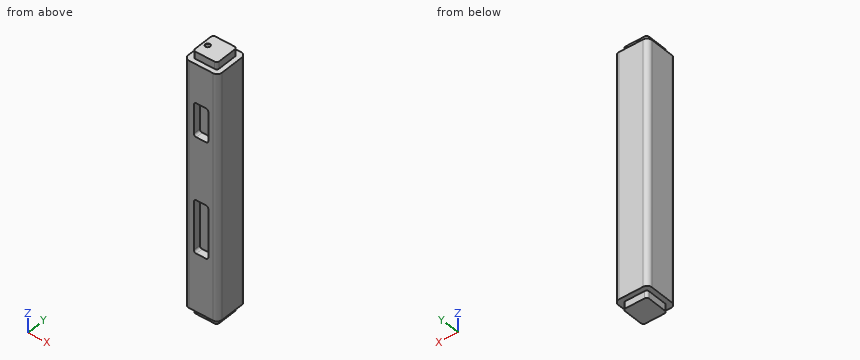
from build123d import *

# Parameters (mm, degrees)
F2_DEPTH  = 647.7
F4_DEPTH  = 19.05
F5_R      = 12.7
F6_R      = 6.35
F7_W      = 38.1
F7_H      = 139.7
F8_DEPTH  = 19.05
F9_R      = 6.35
F11_DEPTH = 19.05
F13_DEPTH = 19.05
F14_R     = 6.35
F15_DEPTH = 2.54


with BuildPart() as f2:
    # F1 (on Top) → F2 (new body)
    with BuildSketch(Plane.XY):
        Polygon((-44.45, 19.05), (-44.45, 0), (-44.45, -19.05), (-44.45, -44.45), (-19.05, -44.45), (0, -44.45), (19.05, -44.45), (44.45, -44.45), (44.45, -19.05), (44.45, 0), (44.45, 19.05), (44.45, 44.45), (19.05, 44.45), (0, 44.45), (-19.05, 44.45), (-44.45, 44.45), align=None)
    extrude(amount=-F2_DEPTH)

    # F3 (on face) → F4 (cut)
    with BuildSketch(Plane.XZ.offset(44.45)):
        Polygon((19.05, -101.6), (-19.05, -101.6), (-19.05, -190.5), (0, -190.5), (19.05, -190.5), align=None)
    extrude(amount=-F4_DEPTH, mode=Mode.SUBTRACT)

    # F5
    f5_edges = [f2.edges().sort_by_distance(p)[0] for p in [
        (-44.45, -44.45, -323.85),
        (44.45, -44.45, -323.85),
        (44.45, 44.45, -323.85),
        (-44.45, 44.45, -323.85),
    ]]
    fillet(f5_edges, radius=F5_R)

    # F6
    f6_edges = [f2.edges().sort_by_distance(p)[0] for p in [
        (-19.05, -34.925, -190.5),
        (19.05, -34.925, -190.5),
        (-19.05, -34.925, -101.6),
        (19.05, -34.925, -101.6),
    ]]
    fillet(f6_edges, radius=F6_R)

    # F7 (on face) → F8 (cut)
    with BuildSketch(Plane.XZ.offset(44.45)):
        with Locations((0, -425.45)):
            Rectangle(F7_W, F7_H)
    extrude(amount=-F8_DEPTH, mode=Mode.SUBTRACT)

    # F9
    f9_edges = [f2.edges().sort_by_distance(p)[0] for p in [
        (-19.05, -34.925, -355.6),
        (19.05, -34.925, -355.6),
        (19.05, -34.925, -495.3),
        (-19.05, -34.925, -495.3),
    ]]
    fillet(f9_edges, radius=F9_R)

    # F10 (on face) → F11 (join)
    with BuildSketch(Plane.XY):
        with BuildLine():
            Line((-25.4, -31.75), (25.4, -31.75))
            ThreePointArc((25.4, -31.75), (29.8901280605, -29.8901280605), (31.75, -25.4))
            Line((31.75, -25.4), (31.75, 25.4))
            ThreePointArc((31.75, 25.4), (29.8901280605, 29.8901280605), (25.4, 31.75))
            Line((25.4, 31.75), (-25.4, 31.75))
            ThreePointArc((-25.4, 31.75), (-29.8901280605, 29.8901280605), (-31.75, 25.4))
            Line((-31.75, 25.4), (-31.75, -25.4))
            ThreePointArc((-31.75, -25.4), (-29.8901280605, -29.8901280605), (-25.4, -31.75))
        make_face()
    extrude(amount=F11_DEPTH)

    # F12 (on face) → F13 (join)
    with BuildSketch(Plane(origin=(0, 0, -647.7), x_dir=(1, 0, 0), z_dir=(0, 0, -1))):
        with BuildLine():
            Line((-25.4, -31.75), (25.4, -31.75))
            ThreePointArc((25.4, -31.75), (29.8901280605, -29.8901280605), (31.75, -25.4))
            Line((31.75, -25.4), (31.75, 25.4))
            ThreePointArc((31.75, 25.4), (29.8901280605, 29.8901280605), (25.4, 31.75))
            Line((25.4, 31.75), (-25.4, 31.75))
            ThreePointArc((-25.4, 31.75), (-29.8901280605, 29.8901280605), (-31.75, 25.4))
            Line((-31.75, 25.4), (-31.75, -25.4))
            ThreePointArc((-31.75, -25.4), (-29.8901280605, -29.8901280605), (-25.4, -31.75))
        make_face()
    extrude(amount=F13_DEPTH)

    # F14 (on face) → F15 (cut)
    with BuildSketch(Plane.XY.offset(19.05)):
        with Locations((-19.05, 0)):
            Circle(F14_R)
    extrude(amount=-F15_DEPTH, mode=Mode.SUBTRACT)


solid = f2.part
Part model, mm, in its own coordinate system. Coordinates: 2 decimals unless noted, no trailing zeros. Loops run counter-clockwise (first coordinate to the right, second up) from the corner with the lowest first, then second, coordinate; pieces in that order, holes last. Notation, with made-up numbers: M 3.5,4.25 L 56.5,4.25 A23 ccw 56.5,38.25 Z; hole C 79.5,-23 d8. An arc over 180 degrees is marked long. Use a Markdown table: item, result. Add a question column.
Q1. Probe L1, parallel to Z at x = 8.5, y = -40; L2, parallel to Y at x = -19.05, z = 17; L3, parallel to Z at x = 31, y = -33. List the from-to ranges inside material, lowest first.
Q2. Cut at A-A (z = -572). Write the cut outline in (x, y), and give its area (3 significant figures).
Q3. Pin check, flat tips, straight feed: P1, Ø15, axis at x = 0, y = -36, coming from the -Z side; P2, Ø5.5, axis at x = 7, z = -660.5, coming from the +Y side; P3, Ø15, axis at x = -10.5, z = -659.5, coming from the -Y side; P4, Ø19, axis at x = -8.5, z = -133.5, coming from the -Y side. Stop position of each tip, or through.
Q4. Cut at D-D (z = -447). Write the cut outline in (x, y).
Q5. Cut at B-B (x = -1). Write the cut outline in (y, z).
Q6. Cut at C-C (y = 0). Write the cut outline in (x, z), and give its area (3 significant figures).
Worked out:
| question | item | result |
|---|---|---|
| 1 | L1 | z = -647.7 to -495.3, -355.6 to -190.5, -101.6 to 0 |
| 1 | L2 | y = -31.75 to -6.35, 6.35 to 31.75 |
| 1 | L3 | z = -647.7 to 0 |
| 2 | outline | M -44.45,-31.75 A12.7 ccw -31.75,-44.45 L 31.75,-44.45 A12.7 ccw 44.45,-31.75 L 44.45,31.75 A12.7 ccw 31.75,44.45 L -31.75,44.45 A12.7 ccw -44.45,31.75 Z |
| 2 | area | 7,760 mm2 |
| 3 | P1 | stops at z = -666.75 |
| 3 | P2 | stops at y = 31.75 |
| 3 | P3 | stops at y = -31.75 |
| 3 | P4 | stops at y = -25.4 |
| 4 | outline | M -44.45,-31.75 A12.7 ccw -31.75,-44.45 L -19.05,-44.45 L -19.05,-25.4 L 19.05,-25.4 L 19.05,-44.45 L 31.75,-44.45 A12.7 ccw 44.45,-31.75 L 44.45,31.75 A12.7 ccw 31.75,44.45 L -31.75,44.45 A12.7 ccw -44.45,31.75 Z |
| 5 | outline | M -44.45,-647.7 L -31.75,-647.7 L -31.75,-666.75 L 31.75,-666.75 L 31.75,-647.7 L 44.45,-647.7 L 44.45,0 L 31.75,0 L 31.75,19.05 L -31.75,19.05 L -31.75,0 L -44.45,0 L -44.45,-101.6 L -25.4,-101.6 L -25.4,-190.5 L -44.45,-190.5 L -44.45,-355.6 L -25.4,-355.6 L -25.4,-495.3 L -44.45,-495.3 Z |
| 6 | outline | M -44.45,-647.7 L -31.75,-647.7 L -31.75,-666.75 L 31.75,-666.75 L 31.75,-647.7 L 44.45,-647.7 L 44.45,0 L 31.75,0 L 31.75,19.05 L -12.7,19.05 L -12.7,16.51 L -25.4,16.51 L -25.4,19.05 L -31.75,19.05 L -31.75,0 L -44.45,0 Z |
| 6 | area | 60,000 mm2 |
